Read the model definition and answer for the solid it produces. Units are mm, in the model's axes. Face numbers are marked on the shaded views. A direction names the side the tool comes from. Coordinates: 2 decimals unless noted, no trailing zeros. Write each loop counter-clockwise with the first axis right and the second up, starting at its lowest first coordinate (ties: lowest second). Pieces come first, ordered by that corner, then holes.
(1) Find the intervals of material crossed by probe 1 along Y at (x, z) = (32, 2.3); probe 2 along X at (y, z) = (7.75, 2.2); probe 3 along X at (y, z) = (10.5, 1.25), in increasing order.
(2) Section C-C on z = 2 is taken. Write down the section's boundary in (x, y).
(3) Section D-D on y = 14 is taken. Write down the section's boundary in (x, z).
(4) Given pin 1 (1.5 mm diameter, centred on x = 52, y = 6.5, fed in from +Z); pin 2 (3.5 mm diameter, centred on x = 7.65, y = 7.9, fed in from +Z), each flat-ended and moving along its own axis, determine where each tip first touches the part or whether it passes through.
(5) Section A-A on x = 28 is taken. Write down the section's boundary in (y, z).
(6) Section B-B on y = 6.5 is taken. Write down the section's boundary in (x, z), then the cut area to 3 significant figures.
(7) Which of the six approach directions +Z, -Z, +X, -X, +Y, -Y give full straight-line access (tool end or side, diameter ignored) to the marked faces 1 and 2?
(8) The mould has two halves that part along X. Classify the marked faces 3, 4 and 5: +X half, -X half, draft (parallel to the pull), parting line (faces both ways), or undercut.
Autodesk Inventor part; units mm, degrees
ref_plane "YZ Plane" through (0, 0, 0) normal (1, 0, 0) x (0, 1, 0)
ref_plane "XZ Plane" through (0, 0, 0) normal (0, 1, 0) x (-1, 0, 0)
ref_plane "XY Plane" through (0, 0, 0) normal (0, 0, 1) x (1, 0, 0)
sketch "Náčrt1" plane through (0, 0, 0) normal (0, 0, 1) x (1, 0, 0)
  line L0 (30.6144, 11.0767) -> (33.1544, 11.0767)
  line L1 (33.1544, 11.0767) -> (25.6544, 11.0767)
  line L2 (25.6544, 11.0767) -> (25.6544, 4.7267)
  line L3 (25.6544, 4.7267) -> (33.1544, 4.7267)
  line L4 (33.1544, 4.7267) -> (33.1544, 11.0767)
  line L5 (58.7544, 14.9017) -> (2.1544, 14.9017)
  circle A0 centre (7.6544, 7.9017) radius 2.25
  line L6 (2.1544, 14.9017) -> (2.1544, 0.9017)
  circle A1 centre (53.2544, 7.9017) radius 2.25
  line L7 (2.1544, 0.9017) -> (58.7544, 0.9017)
  line L8 (58.7544, 0.9017) -> (58.7544, 14.9017)
  point P0 (33.1544, 4.7267)
  point P1 (7.6544, 7.9017)
  point P2 (53.2544, 7.9017)
  dimension "d2" = 7.5
  dimension "d3" = 6.35
extrude "Vysunutí1" add sketch "Náčrt1" along normal blind 4
fillet "Zaoblení1" radius 4 4 edges at (58.7544, 0.9017, 2) (58.7544, 14.9017, 2) (2.1544, 14.9017, 2) (2.1544, 0.9017, 2)
properties part number "Spojovaci_clen"
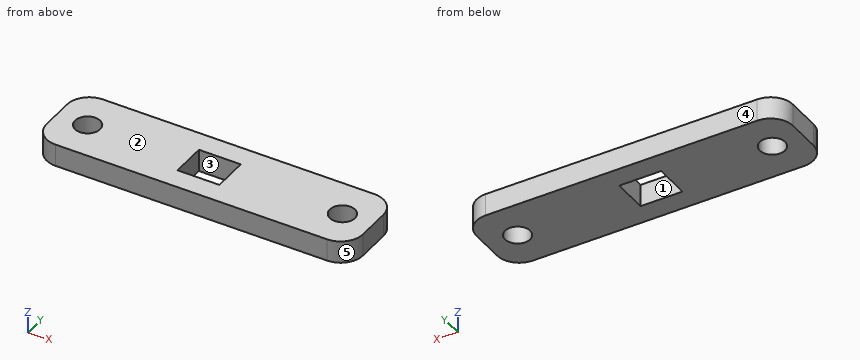
Response:
1. probe 1: y = 0.9 to 4.73, 11.08 to 14.9
1. probe 2: x = 2.15 to 5.41, 9.9 to 25.65, 33.15 to 51.01, 55.5 to 58.75
1. probe 3: x = 2.15 to 25.65, 33.15 to 58.75
2. outline: (2.15, 4.9) arc R4 ccw to (6.15, 0.9) - (54.75, 0.9) arc R4 ccw to (58.75, 4.9) - (58.75, 10.9) arc R4 ccw to (54.75, 14.9) - (6.15, 14.9) arc R4 ccw to (2.15, 10.9) - close; hole circle Ø4.5 at (7.65, 7.9); hole (25.65, 4.73) - (33.15, 4.73) - (33.15, 11.08) - (25.65, 11.08) - close; hole circle Ø4.5 at (53.25, 7.9)
3. outline: (3.62, 0) - (57.28, 0) - (57.28, 4) - (3.62, 4) - close
4. pin 1: stops at z = 4
4. pin 2: passes through
5. outline: (0.9, 0) - (4.73, 0) - (4.73, 4) - (0.9, 4) - close; (11.08, 0) - (14.9, 0) - (14.9, 4) - (11.08, 4) - close
6. outline: (2.15, 0) - (5.89, 0) - (5.89, 4) - (2.15, 4) - close; (9.41, 0) - (25.65, 0) - (25.65, 4) - (9.41, 4) - close; (33.15, 0) - (51.49, 0) - (51.49, 4) - (33.15, 4) - close; (55.01, 0) - (58.75, 0) - (58.75, 4) - (55.01, 4) - close
6. area: 168 mm2
7. face 1: +Z, -Z
7. face 2: +Z, +X, -X, +Y, -Y
8. face 3: undercut
8. face 4: draft
8. face 5: +X half
